Here's how the part is built. I have some questions about the finished solid (model axes, mm). A direction names the side the tool comes from. Coordinates: 2 decimals unless noted, no trailing zeros. Order: outer loops, then holes, each group sorted by start corner. A loop starts at its lowest first (then second) coordinate and runs counter-clockwise, first axis right, second up. Notation, with made-up numbers: (67.25, 41) - (75.25, 41) arc R34 ccw to (75.25, 79) - close; hole circle Ø2 at (3.5, -7). An arc over 180 degrees is marked (long way). Use CSV: the item, a comma, the result in double quotes. Start each with the question number.
from build123d import *

# Parameters (mm, degrees)
SKETCH_1_W      = 23
SKETCH_1_H      = 213.5
SKETCH_1_R      = 1.6
EXTRUDE_1_DEPTH = 4
SKETCH_2_W      = 23
SKETCH_2_H      = 213.5
SKETCH_2_W_2    = 15.3
SKETCH_2_H_2    = 205.8
EXTRUDE_2_DEPTH = 7
CHAMFER_1_SIZE  = 2


with BuildPart() as part:
    # ｽｹｯﾁ1 → ﾎﾞｽ - 押し出し1 (new body)
    with BuildSketch(Plane.XY.offset(5)):
        with Locations((0, -7.25)):
            Rectangle(SKETCH_1_W, SKETCH_1_H)
        with Locations((0, -105)):
            Circle(SKETCH_1_R, mode=Mode.SUBTRACT)
        with Locations((0, -85)):
            Circle(SKETCH_1_R, mode=Mode.SUBTRACT)
        with Locations((0, 90.5)):
            Circle(SKETCH_1_R, mode=Mode.SUBTRACT)
        with Locations((0, 76.66)):
            Circle(SKETCH_1_R, mode=Mode.SUBTRACT)
        with Locations((0, 56.66)):
            Circle(SKETCH_1_R, mode=Mode.SUBTRACT)
        with Locations((0, 29.6)):
            Circle(SKETCH_1_R, mode=Mode.SUBTRACT)
        with Locations((0, 9.6)):
            Circle(SKETCH_1_R, mode=Mode.SUBTRACT)
    extrude(amount=EXTRUDE_1_DEPTH)

    # ｽｹｯﾁ2 → ﾎﾞｽ - 押し出し2 (add)
    with BuildSketch(Plane(origin=(0, 0, 5), x_dir=(-1, 0, 0), z_dir=(0, 0, -1))):
        with Locations((0, -7.25)):
            Rectangle(SKETCH_2_W, SKETCH_2_H)
        with Locations((0, -7.25)):
            Rectangle(SKETCH_2_W_2, SKETCH_2_H_2, mode=Mode.SUBTRACT)
    extrude(amount=EXTRUDE_2_DEPTH)

    # 面取り1
    chamfer_1_edges = [part.edges().sort_by_distance(p)[0] for p in [
        (0, -110.15, -2),
        (-7.65, -7.25, -2),
        (0, 95.65, -2),
        (7.65, -7.25, -2),
    ]]
    chamfer(chamfer_1_edges, length=CHAMFER_1_SIZE)


solid = part.part
Item 1: Suppose I cut it at A-A on y = -53. Write out the boundary of the cut face in (x, z), then the cut area to 3 significant figures.
Item 2: For pin 1 Ø4 at (x, y) = (0, -105) entering from -Z; pin 2 Ø12 at (x, y) = (-2, -35.5) entering from -Z; pin 3 Ø5 at (x, y) = (-6, 58) entering from -Z; pin 4 Ø3.5 at (x, y) = (0, 29.6) entering from +Z, each with a flat end and sliding along its axis, tell me the tip position at first contact or that it passes through.
Item 3: For faces 5 (the flat face through (10, -7, -2)), 6 (the flat face through (-7.65, -9, 3)), which set-ups out of +Z, -Z, +X, -X, +Y, -Y let a thin tool reach every point of the face, with its end or its side?
Item 4: Please list where these lines run through material, in increasing order: line 1 along Y through (x, z) = (3.75, 3.25); line 2 along X through (y, z) = (-80.5, 0.25); line 3 along X through (y, z) = (90.5, 6.55). Write a range as from..to.
Item 5: We'd pull the mould along Y, two halves only. Please class faces 1 (the flat face through (0, 95.65, 3)), 2 (the flat face through (11.5, -9, 4)), 3 (the flat face through (0, 99.5, 4)), 4 (the flat face through (7.65, -9, 3)): released by +Y, released by -Y, zero draft, split by the parting line, or undercut.
Here are the results:
1,outline,"(-11.5, -2) - (-9.65, -2) - (-7.65, 0) - (-7.65, 5) - (7.65, 5) - (7.65, 0) - (9.65, -2) - (11.5, -2) - (11.5, 9) - (-11.5, 9) - close"
1,area,"142 mm^2"
2,pin 1,"z = 5"
2,pin 2,"z = -0.35"
2,pin 3,"z = -0.85"
2,pin 4,"z = 9"
3,face 5,"-Z, +X, -X, +Y, -Y"
3,face 6,"-Z"
4,line 1,"-114..-110.15, 95.65..99.5"
4,line 2,"-11.5..-7.65, 7.65..11.5"
4,line 3,"-11.5..-1.6, 1.6..11.5"
5,face 1,"undercut"
5,face 2,"zero draft"
5,face 3,"released by +Y"
5,face 4,"undercut"
